The model under review builds one solid part; all positions refer to its coordinate system, in mm. A direction names the side the tool comes from. Round coordinates to 2 decimals unless told otherwise and drop trailing zeros. Order: outer loops, then holes, each group sorted by start corner. A loop starts at its lowest first (then second) coordinate and runs counter-clockwise, first axis right, second up. Notation, with made-up numbers: M 61.25,-10.5 L 89.25,-10.5 A33 cw 89.25,22.5 Z; hole C 18,65.5 d10. An arc over 180 degrees is marked long. Answer as a JSON object with one key per item and string values. Group by question number.
1) For faces 1 (the cylindrical face through (-19.57, -18.82, 10.29)), 2 (the conical face through (-9.7, -3.8, 10.1)), 3 (the flat face through (-9, 16, 10)), list the 3-axis set-ups (+Z, -Z, +X, -X, +Y, -Y) from which the entire face can be reached by the end or side of a thin tool; tool diameter is ignored.
2) To check wall thickness, follow line 1 (Y direction, x = -22.25, z = 10.5); line 2 (Z direction, x = -28.75, y = 0); line 3 (X direction, y = -4.5, z = 4). State the ranges of each line that lie inside material, in increasing order.
3) Consider section A-A, the plane x = -27.5. Write out the cut boundary in (y, z), then the cut area to 3 significant figures.
4) Consider section D-D, the plane z = 2.5. Write out the cut boundary in (x, y), then the cut area to 3 significant figures.
5) The part is to be moulded in two halves that separate along Z. For faces 4 (the flat face through (-9, -16, 10)), 5 (the flat face through (-10, 0, 24.5)), 6 (the cylindrical face through (-14.44, -1.05, 7.46)), say which applies: +Z half, -Z half, draft (parallel to the pull), parting line (faces both ways), or undercut.
6) Insertion check: pin 1 Ø5 at (y, z) = (11, 11) entering from +X; pin 2 Ø9.5 at (x, y) = (-24, 9.5) entering from -Z; pin 3 Ø11.5 at (x, y) = (-24.5, -20) entering from +Z; pin 4 Ø4 at (x, y) = (-24.82, -19.05) entering from +Z. Each pin has a flat end and moves straight along its axis. Give the tip position at first contact, or say it passes through.
```python
from build123d import *

# Parameters (mm, degrees)
SKETCH1_W           = 20.861
SKETCH1_H           = 57.912
SKETCH1_R           = 3.25
BOSS_EXTRUDE1_DEPTH = 6
BOSS_EXTRUDE2_DEPTH = 57.912
SKETCH8_R           = 3.25
CUT_EXTRUDE4_DEPTH  = 49.898888096
CUT_EXTRUDE5_START  = -6
SKETCH9_R           = 5.25
CUT_EXTRUDE5_DEPTH  = 43.898888096
SKETCH10_R          = 2.75
CUT_EXTRUDE6_DEPTH  = 44.28835013
CUT_EXTRUDE7_START  = -9
SKETCH11_R          = 5.25
CUT_EXTRUDE7_DEPTH  = 35.28835013
SKETCH12_W          = 12
SKETCH12_H          = 0.35
CUT_EXTRUDE8_DEPTH  = 71.046063879
FILLET1_R           = 4
BOSS_EXTRUDE3_START = 1
SKETCH13_W          = 6
SKETCH13_H          = 57.912
SKETCH13_R          = 2.75
BOSS_EXTRUDE3_DEPTH = 1
CHAMFER1_SIZE       = 2.5
SKETCH14_R          = 3.5
CUT_EXTRUDE9_DEPTH  = 1
CHAMFER2_SIZE       = 1


# Some blends are built 0.0001 mm under size
with BuildPart() as part:
    # Sketch1 → Boss-Extrude1 (new body)
    # profile 1 of 3: a face of its own
    with BuildSketch(Plane.XY):
        with Locations((-20.4305, 0)):
            Rectangle(SKETCH1_W, SKETCH1_H)
        with Locations((-24.8158, 19.05)):
            Circle(SKETCH1_R, mode=Mode.SUBTRACT)
        with Locations((-24.8158, -19.05)):
            Circle(SKETCH1_R, mode=Mode.SUBTRACT)
    # profile 2 of 3: a face of its own
    with BuildSketch(Plane.XY):
        with Locations((-24.8158, 19.05)):
            Circle(SKETCH1_R)
    # profile 3 of 3: a face of its own
    with BuildSketch(Plane.XY):
        with Locations((-24.8158, -19.05)):
            Circle(SKETCH1_R)
    extrude(amount=BOSS_EXTRUDE1_DEPTH)

    # Sketch7 → Boss-Extrude2 (add)
    with BuildSketch(Plane.XZ.offset(28.956)):
        Polygon((-30.861, 6), (-16, 20.5), (-16, 24.5), (-8.9, 24.5), (-8.9, 20.5), (-10, 20.5), (-10, 6), align=None)
    extrude(amount=-BOSS_EXTRUDE2_DEPTH)

    # Sketch8 → Cut-Extrude4 (cut, through all)
    with BuildSketch(Plane(origin=(0, 0, 0), x_dir=(-1, 0, 0), z_dir=(0, 0, -1))):
        with Locations((24.8158, -19.05)):
            Circle(SKETCH8_R)
        with Locations((24.8158, 19.05)):
            Circle(SKETCH8_R)
    extrude(amount=-CUT_EXTRUDE4_DEPTH, mode=Mode.SUBTRACT)

    # Sketch9 → Cut-Extrude5 (cut, through all)
    with BuildSketch(Plane(origin=(0, 0, 0), x_dir=(-1, 0, 0), z_dir=(0, 0, -1)).offset(CUT_EXTRUDE5_START)):
        with Locations((24.8158, -19.05)):
            Circle(SKETCH9_R)
        with Locations((24.8158, 19.05)):
            Circle(SKETCH9_R)
    extrude(amount=-CUT_EXTRUDE5_DEPTH, mode=Mode.SUBTRACT)

    # Sketch10 → Cut-Extrude6 (cut, through all)
    with BuildSketch(Plane(origin=(-10, 0, 0), x_dir=(0, 0, -1), z_dir=(1, 0, 0))):
        with Locations((-10, 0)):
            Circle(SKETCH10_R)
    extrude(amount=-CUT_EXTRUDE6_DEPTH, mode=Mode.SUBTRACT)

    # Sketch11 → Cut-Extrude7 (cut, through all)
    with BuildSketch(Plane(origin=(-10, 0, 0), x_dir=(0, 0, -1), z_dir=(1, 0, 0)).offset(CUT_EXTRUDE7_START)):
        with Locations((-10, 0)):
            Circle(SKETCH11_R)
    extrude(amount=-CUT_EXTRUDE7_DEPTH, mode=Mode.SUBTRACT)

    # Sketch12 → Cut-Extrude8 (cut, through all)
    with BuildSketch(Plane(origin=(0, 28.956, 0), x_dir=(1, 0, 0), z_dir=(0, 1, 0))):
        with Locations((-24.861, -0.175)):
            Rectangle(SKETCH12_W, SKETCH12_H)
    extrude(amount=-CUT_EXTRUDE8_DEPTH, mode=Mode.SUBTRACT)

    # Fillet1
    fillet1_edges = [part.edges().sort_by_distance(p)[0] for p in [
        (-16, 0, 24.5),
    ]]
    fillet(fillet1_edges, radius=FILLET1_R - 0.0001)  # a hair under: the kernel refuses the full size

    # Sketch13 → Boss-Extrude3 (add)
    with BuildSketch(Plane(origin=(-10, 0, 0), x_dir=(0, 0, -1), z_dir=(1, 0, 0)).offset(BOSS_EXTRUDE3_START)):
        with Locations((-10, 0)):
            Rectangle(SKETCH13_W, SKETCH13_H)
        with Locations((-10, 0)):
            Circle(SKETCH13_R, mode=Mode.SUBTRACT)
    extrude(amount=-BOSS_EXTRUDE3_DEPTH)

    # Chamfer1
    # the kernel refuses this chamfer: 2.5 mm, written as the material it adds along each edge
    with BuildSketch(Plane(origin=(-19, 0, 10), x_dir=(0, 0, -1), z_dir=(0, -1, 0))) as chamfer1_piece_1_section:
        Polygon((5.25 - CHAMFER1_SIZE, 0), (5.25, -CHAMFER1_SIZE), (5.25, 0), align=None)
    chamfer1_piece_1 = revolve(axis=Axis((-19, 0, 10), (1, 0, 0)), mode=Mode.PRIVATE)
    chamfer1_piece_1 = chamfer1_piece_1 - Plane(origin=(-20.253037954, 0, 10), x_dir=(0, 0, -1), z_dir=(1, 0, 0)) * Cylinder(2.75, 21, mode=Mode.PRIVATE)
    chamfer1_piece_1 = split(chamfer1_piece_1, bisect_by=Plane(origin=(-21.393994511, 0, 15.237035166), z_dir=(0.6983599622441906, 0, -0.7157467171662703)), keep=Keep.TOP, mode=Mode.PRIVATE)
    add(chamfer1_piece_1)

    # Sketch14 → Cut-Extrude9 (cut)
    with BuildSketch(Plane(origin=(-9, 0, 0), x_dir=(0, 0, -1), z_dir=(1, 0, 0))):
        with Locations((-10, 0)):
            Circle(SKETCH14_R)
    extrude(amount=-CUT_EXTRUDE9_DEPTH, mode=Mode.SUBTRACT)

    # Chamfer2
    chamfer2_edges = [part.edges().sort_by_distance(p)[0] for p in [
        (-9, -3.5, 10),
        (-9, 3.5, 10),
    ]]
    chamfer(chamfer2_edges, length=CHAMFER2_SIZE - 0.0001)  # a hair under: the kernel refuses the full size


solid = part.part
```
Results list:
{
 "1": {"face 1": "+Z", "face 2": "+X", "face 3": "-Z, +X, +Y, -Y"},
 "2": {"line 1": "-28.96 to -23.63, -14.47 to -5.23, 5.23 to 14.47, 23.63 to 28.96", "line 2": "0.35 to 4.75", "line 3": "-30.86 to -10"},
 "3": {"outline": "M -28.96,0.35 L -20.88,0.35 L -20.88,6 L -23.56,6 L -23.56,9.28 L -28.96,9.28 Z; M -17.22,0.35 L 17.22,0.35 L 17.22,6 L 14.54,6 L 14.54,9.28 L 5.2,9.28 A5.25 cw -5.2,9.28 L -14.54,9.28 L -14.54,6 L -17.22,6 Z; M 20.88,0.35 L 28.96,0.35 L 28.96,9.28 L 23.56,9.28 L 23.56,6 L 20.88,6 Z", "area": "381 mm^2"},
 "4": {"outline": "M -30.86,-28.96 L -10,-28.96 L -10,28.96 L -30.86,28.96 Z; hole C -24.82,-19.05 d6.5; hole C -24.82,19.05 d6.5", "area": "1,140 mm^2"},
 "5": {"face 4": "draft", "face 5": "+Z half", "face 6": "undercut"},
 "6": {"pin 1": "x = -9", "pin 2": "z = 0.35", "pin 3": "z = 17.82", "pin 4": "through"}
}
